from build123d import *

# Parameters (mm, degrees)
BOSS_EXTRUDE1_DEPTH = 20
SKETCH2_R           = 5.612511992
BOSS_EXTRUDE2_DEPTH = 262
SKETCH3_R           = 3.25
CUT_EXTRUDE1_DEPTH  = 10
SKETCH4_R           = 3.25
CUT_EXTRUDE2_DEPTH  = 10


with BuildPart() as part:
    # Sketch1 → Boss-Extrude1 (new body)
    with BuildSketch(Plane.XY):
        Polygon((-75, -125), (-75, 125), (-75, 130), (-63.356925632, 130), (75, 130), (75, 125), (75, -125), (75, -130), (-75, -130), align=None)
        Polygon((-55, -105), (-55, 105), (-55, 125), (55, 125), (55, 105), (55, -105), (55, -125), (-55, -125), align=None, mode=Mode.SUBTRACT)
    extrude(amount=BOSS_EXTRUDE1_DEPTH)

    # Sketch2 → Boss-Extrude2 (add)
    with BuildSketch(Plane.XZ.offset(130)):
        with Locations(Location((-28, 10, 0), (0, 0, 90))):
            Circle(SKETCH2_R)
        with Locations(Location((28, 10, 0), (0, 0, 90))):
            Circle(SKETCH2_R)
    extrude(amount=-BOSS_EXTRUDE2_DEPTH)

    # Sketch3 → Cut-Extrude1 (cut)
    with BuildSketch(Plane.XZ.offset(-125)):
        with Locations(Location((-44.25, 10, 0), (0, 0, 270))):
            Circle(SKETCH3_R)
        with Locations(Location((-11.75, 10, 0), (0, 0, 270))):
            Circle(SKETCH3_R)
        with Locations(Location((11.75, 10, 0), (0, 0, 270))):
            Circle(SKETCH3_R)
        with Locations(Location((44.25, 10, 0), (0, 0, 270))):
            Circle(SKETCH3_R)
    extrude(amount=-CUT_EXTRUDE1_DEPTH, mode=Mode.SUBTRACT)

    # Sketch4 → Cut-Extrude2 (cut)
    with BuildSketch(Plane.XZ.offset(130)):
        with Locations(Location((-44.25, 10, 0), (0, 0, 270))):
            Circle(SKETCH4_R)
        with Locations(Location((-11.75, 10, 0), (0, 0, 270))):
            Circle(SKETCH4_R)
        with Locations(Location((11.75, 10, 0), (0, 0, 270))):
            Circle(SKETCH4_R)
        with Locations(Location((44.25, 10, 0), (0, 0, 270))):
            Circle(SKETCH4_R)
    extrude(amount=-CUT_EXTRUDE2_DEPTH, mode=Mode.SUBTRACT)


solid = part.part
Model file for the job. Use its own axes, mm. A direction names the side the tool comes from. Coordinates: 2 decimals unless noted, no trailing zeros. Write each loop counter-clockwise with the first axis right and the second up, starting at its lowest first coordinate (ties: lowest second). Pieces come first, ordered by that corner, then holes. Notation, with made-up numbers: (68.5, 41) -> (91.5, 41) arc R11 cw to (91.5, 61) -> close; hole circle Ø4 at (-1.5, 54). An arc over 180 degrees is marked (long way). One line per item, written item: value. Start each with the question number.
1) Slice it at C-C on z = 10. Count the separate pieces of the cut face and the enclosed holes in it, then the cut area to 3 significant figures.
2) Slice it at B-B on y = -99. Write the cut outline in (x, z), then the cut area to 3 significant figures.
3) Flat gauge pins, fed straight in: pin 1 Ø4 at (x, y) = (31.5, -89) entering from -Z; pin 2 Ø7.5 at (x, z) = (44.25, 10) entering from +Y; pin 3 Ø2 at (x, y) = (35, 58.5) entering from +Z; pin 4 Ø6 at (x, y) = (25.5, 49.5) entering from -Z. Where does each tip first touch, or does it go through?
4) Probe probe 1 along X at (y, z) = (-67, 9.25); probe 2 along X at (y, z) = (-127.1, 10); probe 3 along Y at (x, z) = (37, 12.5). List the from-to ranges inside material, lowest first.
5) Pull direction X, two halves, no side cores. Call faces 1 (the face through (-55.2, 10.2, 0)), 2 (the face through (-75, 2, 10)), 3 (the face through (-23.02, 130.99, 12.59)): +X half, -X half, draft (parallel to the pull), parting line (faces both ways), or undercut.
6) Which spindle directions (+Z, -Z, +X, -X, +Y, -Y) get a long thin tool onto all of the face, cutting with end or side? Do faces 4 (the face through (32.98, 130.99, 12.59)), 5 (the face through (32.98, -1.75, 12.59)), 6 (the face through (-55, -2, 10)). Say none if no direction does.
7) Slice it at A-A on x = 11.75. Write the cut outline in (y, z).
Answers follow:
1. separate pieces: 6
1. enclosed holes: 0
1. area: 16,900 mm2
2. outline: (-75, 0) -> (-55, 0) -> (-55, 20) -> (-75, 20) -> close; circle Ø11.23 at (-28, 10); circle Ø11.23 at (28, 10); (55, 0) -> (75, 0) -> (75, 20) -> (55, 20) -> close
2. area: 998 mm2
3. pin 1: z = 4.59
3. pin 2: y = 130
3. pin 3: through
3. pin 4: z = 4.39
4. probe 1: -75 to -55, -33.56 to -22.44, 22.44 to 33.56, 55 to 75
4. probe 2: -75 to -47.5, -41 to -15, -8.5 to 8.5, 15 to 41, 47.5 to 75
4. probe 3: -130 to -125, 125 to 130
5. face 1: draft
5. face 2: -X half
5. face 3: undercut
6. face 4: +Y
6. face 5: none
6. face 6: +Z, -Z
7. outline: (-130, 0) -> (-125, 0) -> (-125, 6.75) -> (-130, 6.75) -> close; (-130, 13.25) -> (-125, 13.25) -> (-125, 20) -> (-130, 20) -> close; (125, 0) -> (130, 0) -> (130, 6.75) -> (125, 6.75) -> close; (125, 13.25) -> (130, 13.25) -> (130, 20) -> (125, 20) -> close
